```python
from build123d import *

# Parameters (mm, degrees)
SKETCH1_W           = 500
SKETCH1_H           = 250
BOSS_EXTRUDE1_DEPTH = 10
SKETCH2_R           = 25
SKETCH2_R_2         = 12.5
BOSS_EXTRUDE2_DEPTH = 100


with BuildPart() as part:
    # Sketch1 → Boss-Extrude1 (new body)
    with BuildSketch(Plane.XY):
        Rectangle(SKETCH1_W, SKETCH1_H)
    extrude(amount=BOSS_EXTRUDE1_DEPTH)

    # Sketch2 → Boss-Extrude2 (add)
    with BuildSketch(Plane.XY.offset(10)):
        with Locations(Location((-140, 0, 0), (0, 0, 180))):
            Circle(SKETCH2_R)
        with Locations(Location((140, 0, 0), (0, 0, 180))):
            Circle(SKETCH2_R_2)
    extrude(amount=BOSS_EXTRUDE2_DEPTH)


solid = part.part
```
Can you work these out from the model? Positions are in its coordinate system, mm. A direction names the side the tool comes from. Give positions to 0.01 mm unless a question says otherwise; leave off trailing zeros. Order: outer loops, then holes, each group sorted by start corner. A loop starts at its lowest first (then second) coordinate and runs counter-clockwise, first axis right, second up. Notation, with made-up numbers: (27, 20) - (51, 20) arc R15 cw to (51, 41) - close; hole circle Ø8 at (-34.75, 3). An arc over 180 degrees is marked (long way). Use a Markdown table: item, result. Add a question column.
Q1. If we section it at A-A on x = -140: Write out the boundary of the cut face in (y, z).
Q2. If we section it at D-D on x = 140: Write out the boundary of the cut face in (y, z).
Q3. If we section it at C-C on z = 16: Write out the boundary of the cut face in (x, y), plus the area to 3 significant figures.
Q4. Please list where these lines run through material, in increasing order: line 1 along Z through (x, y) = (-11, 33); line 2 along X through (y, z) = (4, 55); line 3 along X through (y, z) = (15, 55).
Q5. On a 3-axis mill with a long thin cutter (end or side, diameter ignored), from which of +Z, -Z, +X, -X, +Y, -Y can I reach the whole of each face in a straight line? I mean faces 4 (the flat face through (-140, 0, 110)), 5 (the cylindrical face through (-121.574, -16.896, 59.3)). Say none if no direction works.
Q6. If we mould it in two halves opening along X, with no side actions, what happens to faces 1 (the cylindrical face through (128.077, -3.755, 59.3)), 2 (the flat face through (250, -2, 5)), 3 (the flat face through (-3, 125, 5))? For each: released by +X, released by -X, zero draft, split by the parting line, or undercut.
Q7. I'm going to push flat-ended pins straight in: pin 1 (5 mm diameter, centred on x = -51.5, y = -38.5, fed in from +Z); pin 2 (2 mm diameter, centred on y = -13.5, z = 55, fed in from -X). Where does each tip first touch, or does it pass through?
Q8. If we section it at B-B on y = 0: Write out the boundary of the cut face in (x, z).
Answers follow:
| question | item | result |
|---|---|---|
| 1 | outline | (-125, 0) - (125, 0) - (125, 10) - (25, 10) - (25, 110) - (-25, 110) - (-25, 10) - (-125, 10) - close |
| 2 | outline | (-125, 0) - (125, 0) - (125, 10) - (12.5, 10) - (12.5, 110) - (-12.5, 110) - (-12.5, 10) - (-125, 10) - close |
| 3 | outline | circle Ø50 at (-140, 0); circle Ø25 at (140, 0) |
| 3 | area | 2,450 mm^2 |
| 4 | line 1 | z = 0 to 10 |
| 4 | line 2 | x = -164.68 to -115.32, 128.16 to 151.84 |
| 4 | line 3 | x = -160 to -120 |
| 5 | face 4 | +Z, +X, -X, +Y, -Y |
| 5 | face 5 | +Z |
| 6 | face 1 | undercut |
| 6 | face 2 | released by +X |
| 6 | face 3 | zero draft |
| 7 | pin 1 | stops at z = 10 |
| 7 | pin 2 | stops at x = -161.65 |
| 8 | outline | (-250, 0) - (250, 0) - (250, 10) - (152.5, 10) - (152.5, 110) - (127.5, 110) - (127.5, 10) - (-115, 10) - (-115, 110) - (-165, 110) - (-165, 10) - (-250, 10) - close |
